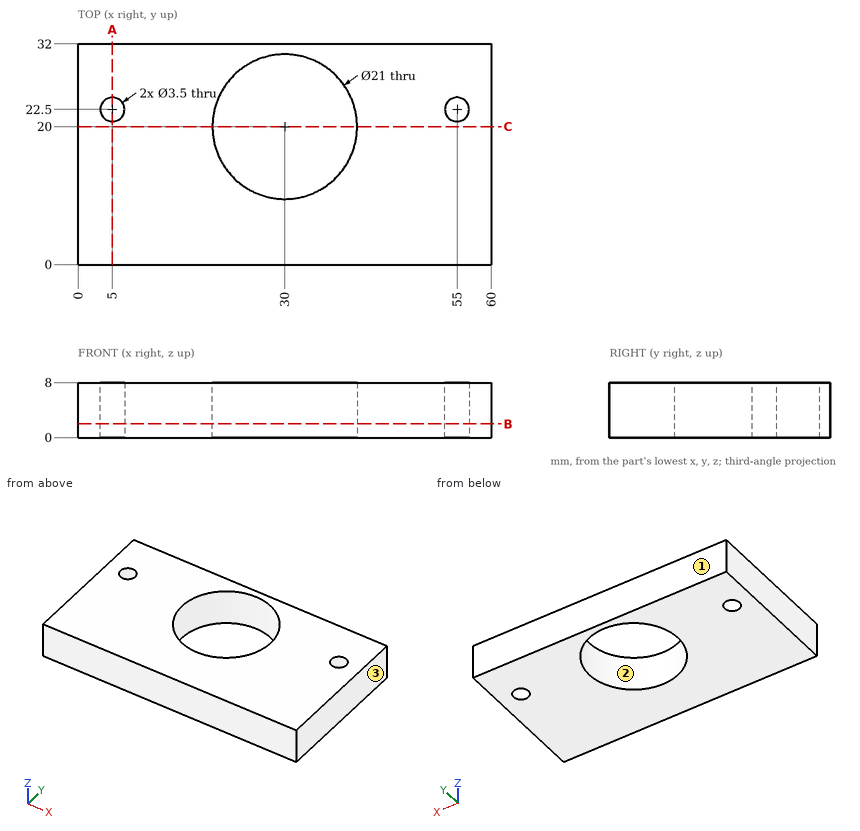
Could you check a few things on this drawing? It's one solid part, dimensions in mm from its lowest x, y, z. Round coordinates to 2 decimals unless told otherwise and drop trailing zeros. Loops run counter-clockwise (first coordinate to the right, second up) from the corner with the lowest first, then second, coordinate; pieces in that order, holes last.
Q1. I want a section at B-B (z = 2). Write out the boundary of the cut face in (x, y).
Q2. I want a section at A-A (x = 5). Write out the boundary of the cut face in (y, z), and give its area (3 significant figures).
Q3. I want a section at C-C (y = 20). Write out the boundary of the cut face in (x, z), and give its area (3 significant figures).
Q4. Thinking about a two-plate mould opening in Y: for the marked faces 1, 2 and 3, which applies, pulls with the +Y half, pulls with the -Y half, needs draft (parallel to the pull), parting line crosses it, or undercut?
Q5. Please list where these lines run through material, in increasing order: L1, parallel to Y at x = 55, z = 3.5; L2, parallel to X at y = 22, z = 2; L3, parallel to X at y = 24, z = 4.5.
Q6. For P1, Ø5.5, axis at x = 5, y = 22.5, coming from the +Z side; P2, Ø2, axis at x = 55, y = 22.5, coming from the +Z side, each with a flat end and sliding along its axis, tell me the tip position at first contact or that it passes through.
Answer below:
1. outline: (0, 0) - (60, 0) - (60, 32) - (0, 32) - close; hole circle Ø3.5 at (5, 22.5); hole circle Ø21 at (30, 20); hole circle Ø3.5 at (55, 22.5)
2. outline: (0, 0) - (20.75, 0) - (20.75, 8) - (0, 8) - close; (24.25, 0) - (32, 0) - (32, 8) - (24.25, 8) - close
2. area: 228 mm2
3. outline: (0, 0) - (19.5, 0) - (19.5, 8) - (0, 8) - close; (40.5, 0) - (60, 0) - (60, 8) - (40.5, 8) - close
3. area: 312 mm2
4. face 1: pulls with the +Y half
4. face 2: undercut
4. face 3: needs draft
5. L1: y = 0 to 20.75, 24.25 to 32
5. L2: x = 0 to 3.32, 6.68 to 19.69, 40.31 to 53.32, 56.68 to 60
5. L3: x = 0 to 4.1, 5.9 to 20.29, 39.71 to 54.1, 55.9 to 60
6. P1: stops at z = 8
6. P2: passes through
